Design review of the part built by this model. Coordinates are the model's own, in mm. A direction names the side the tool comes from. Coordinates: 2 decimals unless noted, no trailing zeros. Write each loop counter-clockwise with the first axis right and the second up, starting at its lowest first coordinate (ties: lowest second). Pieces come first, ordered by that corner, then holes.
Q1. For pin 1 Ø1.5 at (y, z) = (-1, -6.5) entering from -X, flat-tipped, find the tip position at first contact; note if it passes through.
Q2. For faces 5 (the cylindrical face through (-27, 0, 9)), 6 (the flat face through (-10, 0, 0)), list the 3-axis set-ups (+Z, -Z, +X, -X, +Y, -Y) from which the entire face can be reached by the end or side of a thin tool; tool diameter is ignored.
Q3. Take a section at A-A, the plane x = -12.5. Write out the cut boundary in (y, z).
Q4. The part is to be moulded in two halves that separate along X. For faces 1 (the flat face through (21.8, -2.3, -6)), 2 (the cylindrical face through (35, 0, 9)), 3 (the cylindrical face through (-35, 0, -9)), 4 (the cylindrical face through (-27, 0, -9)), say which applies: released by +X, released by -X, zero draft, split by the parting line, or undercut.
Q5. Take a section at C-C, the plane y = -6. Write out the cut boundary in (x, z), plus the area to 3 significant figures.
Q6. Take a section at B-B, the plane z = 0. Write out the cut boundary in (x, y).
Q7. Take a section at D-D, the plane x = 0. Write out the cut boundary in (y, z), plus the area to 3 significant figures.
Q8. For L1, parallel to X at y = 0, z = 9.5; L2, parallel to Y at x = -24, z = -8.85; L3, parallel to Z at x = -25.5, y = -4, list the stretches that pass through material, from the lowest coordinate up.
Autodesk Inventor part; units mm, degrees
ref_plane "Pracovní rovina1" through (0, 0, 6) normal (0, 0, 1) x (1, 0, 0)
ref_plane "YZ Plane" through (0, 0, 0) normal (1, 0, 0) x (0, 1, 0)
ref_plane "XZ Plane" through (0, 0, 0) normal (0, 1, 0) x (-1, 0, 0)
sketch "Náčrt1" plane through (0, 0, 0) normal (0, 0, 1) x (1, 0, 0)
  line L0 (0, -15.4) -> (0, 15.4) construction
  line L1 (-49, 0) -> (49, 0) construction
  arc A0 (-24, 11) -> (-24, -11) centre (-24, 0) ccw
  arc A1 (24, -11) -> (24, 11) centre (24, 0) ccw
  line L2 (-24, 11) -> (24, 11)
  line L3 (-24, -11) -> (24, -11)
  circle A2 centre (-24, 0) radius 3
  circle A3 centre (24, 0) radius 3
  point P0 (0, 0)
  point P1 (0, -11)
  point P2 (0, 11)
  dimension "d0" = 22
  dimension "d1" = 22
  dimension "d2" = 48
  dimension "d3" = 6
  dimension "d4" = 6
extrude "Vysunutí1" add sketch "Náčrt1" along normal mid plane 24
ref_plane "Pracovní rovina1" through (0, 0, 6) normal (0, 0, 1) x (1, 0, 0)
sketch "Náčrt2" plane through (0, 0, 6) normal (0, 0, 1) x (1, 0, 0)
  line L0 (-56, 0) -> (56, 0) construction
  line L1 (0, -15.4) -> (0, 15.4) construction
  line L2 (11, 11) -> (9, -11)
  line L3 (9, -11) -> (40, -11)
  line L4 (40, -11) -> (40, 11)
  line L5 (40, 11) -> (11, 11)
  line L6 (24, 11) -> (-24, 11) construction
  line L7 (-24, -11) -> (24, -11) construction
  line L8 (-11, 11) -> (-9, -11)
  line L9 (-9, -11) -> (-40, -11)
  line L10 (-40, -11) -> (-40, 11)
  line L11 (-40, 11) -> (-11, 11)
  point P0 (0, 0)
  dimension "d10" = 11
  dimension "d11" = 9
  dimension "d12" = 40
  dimension "d15" = 0
  dimension "d16" = 0
extrude "Vysunutí3" cut sketch "Náčrt2" against normal blind 12
sketch "Náčrt3" plane through (-24, 11, -12) normal (0, 1, 0) x (1, 0, 0)
  circle A0 centre (24, -12) radius 6
  dimension "d19" = 12
extrude "Vysunutí4" cut sketch "Náčrt3" against normal up to next
chamfer "Zkosení1" distance 1 angle 45 2 edges at (-6, 11, 0) (-6, -11, 0)
chamfer "Zkosení2" distance 0.5 angle 45 4 edges at (-27, 0, 12) (21, 0, 12) (21, 0, -12) (-27, 0, -12)
thread "Závit1"
properties part number "Součást25"
Responses:
1. pin 1: stops at x = -35
2. face 5: +Z, -Z
2. face 6: -X, -Y
3. outline: (-11, -12) - (11, -12) - (11, -6) - (-11, -6) - close; (-11, 6) - (11, 6) - (11, 12) - (-11, 12) - close
4. face 1: zero draft
4. face 2: released by +X
4. face 3: released by -X
4. face 4: undercut
5. outline: (-33.22, -12) - (33.22, -12) - (33.22, -6) - (9.45, -6) - (9.45, 6) - (33.22, 6) - (33.22, 12) - (-33.22, 12) - (-33.22, 6) - (-9.45, 6) - (-9.45, -6) - (-33.22, -6) - close; hole circle Ø12 at (0, 0)
5. area: 911 mm2
6. outline: (-11, 11) - (-9, -11) - (-7, -11) - (-6, -10) - (-6, 10) - (-7, 11) - close; (6, -10) - (7, -11) - (9, -11) - (11, 11) - (7, 11) - (6, 10) - close
7. outline: (-11, -12) - (11, -12) - (11, -7) - (10, -6) - (-10, -6) - (-11, -7) - close; (-11, 7) - (-10, 6) - (10, 6) - (11, 7) - (11, 12) - (-11, 12) - close
7. area: 262 mm2
8. L1: x = -35 to -27, -21 to 21, 27 to 35
8. L2: y = -11 to -3, 3 to 11
8. L3: z = -12 to -6, 6 to 12
